The listing builds one solid part. Answer for the finished solid, in the listing's coordinates (mm). A direction names the side the tool comes from. Give positions to 0.01 mm unless a question says otherwise; leave off trailing zeros. Order: outer loops, then holes, each group sorted by start corner. A loop starts at its lowest first (then second) coordinate and runs counter-clockwise, first axis right, second up.
```python
from build123d import *

# Parameters (mm, degrees)
SKETCH1_W            = 196
SKETCH1_H            = 46
BOSS_EXTRUDE1_DEPTH  = 3.175
SKETCH2_W            = 30
SKETCH2_H            = 10.018068389
SKETCH2_W_2          = 48.596040924
SKETCH2_H_2          = 27.403064809
CUT_EXTRUDE1_DEPTH   = 3.175
M5_CLEARANCE_HOLE1_D = 5.3


with BuildPart() as part:
    # Sketch1 → Boss-Extrude1 (new body)
    with BuildSketch(Plane(origin=(0, 0, 0), x_dir=(1, 0, 0), z_dir=(0, 1, 0))):
        with Locations((98, 23)):
            Rectangle(SKETCH1_W, SKETCH1_H)
    extrude(amount=BOSS_EXTRUDE1_DEPTH)

    # Sketch2 → Cut-Extrude1 (cut)
    with BuildSketch(Plane(origin=(0, 3.175, 0), x_dir=(1, 0, 0), z_dir=(0, 1, 0))):
        with Locations((98, 40.990965805)):
            Rectangle(SKETCH2_W, SKETCH2_H)
        with BuildLine():
            ThreePointArc((83, 35.981931611), (98, 20.981931611), (113, 35.981931611))
            Line((113, 35.981931611), (83, 35.981931611))
        make_face()
        with Locations((107.298020462, 32.298467596)):
            Rectangle(SKETCH2_W_2, SKETCH2_H_2)
    extrude(amount=-CUT_EXTRUDE1_DEPTH, mode=Mode.SUBTRACT)

    # M5 Clearance Hole1 (through all)
    with Locations(Plane(origin=(0, 3.175, 0), x_dir=(1, 0, 0), z_dir=(0, 1, 0))):
        with Locations((188.5, 10), (7.5, 10), (188.5, 42), (7.5, 42)):
            Hole(M5_CLEARANCE_HOLE1_D / 2)


solid = part.part
```
1) Given P1, Ø1.6, axis at x = 114.5, y = 2.5, coming from the -Z side; P2, Ø7, axis at x = 7.5, z = -10, coming from the -Y side, each flat-ended and moving along its own axis, determine where each tip first touches the part or whether it passes through.
Geometry says:
P1: stops at z = -18.6
P2: stops at y = 0
2) Find section D-D (y = 2.15). Write down the section's boundary in (x, z), then the cut area to 3 significant figures.
Geometry says:
outline: (0, -46) - (83, -46) - (83, -18.6) - (131.6, -18.6) - (131.6, -46) - (196, -46) - (196, 0) - (0, 0) - close; hole circle Ø5.3 at (7.5, -42); hole circle Ø5.3 at (7.5, -10); hole circle Ø5.3 at (188.5, -42); hole circle Ø5.3 at (188.5, -10)
area: 7,600 mm2
3) A tool of negligible diameter and unlimited length cuts with its end or side. For faces 1 (the flat face through (0, 2, -23)), 2 (the flat face through (131.596, 2, -32)), from which of +Z, -Z, +X, -X, +Y, -Y can it reach the whole face along a straight path? Write none if from no direction.
Geometry says:
face 1: +Z, -Z, -X, +Y, -Y
face 2: -Z, +Y, -Y
4) Find section A-A (z = -37.5). Write down the section's boundary in (x, y) (3 decimals), then the cut area to 3 significant figures.
Geometry says:
outline: (0, 0) - (83, 0) - (83, 3.175) - (0, 3.175) - close; (131.596, 0) - (196, 0) - (196, 3.175) - (131.596, 3.175) - close
area: 468 mm2
5) Find section C-C (z = -10). Write down the section's boundary in (x, y) (3 decimals).
Geometry says:
outline: (0, 0) - (4.85, 0) - (4.85, 3.175) - (0, 3.175) - close; (10.15, 0) - (185.85, 0) - (185.85, 3.175) - (10.15, 3.175) - close; (191.15, 0) - (196, 0) - (196, 3.175) - (191.15, 3.175) - close
6) Straight lines are drawn through the part: probe 1 along X at (y, z) = (2.15, -42); probe 2 along Z at (x, y) = (188.5, 2.05); probe 3 along X at (y, z) = (2.45, -10). For each, find the intervals that lie inside material, in ascending order.
Geometry says:
probe 1: x = 0 to 4.85, 10.15 to 83, 131.6 to 185.85, 191.15 to 196
probe 2: z = -46 to -44.65, -39.35 to -12.65, -7.35 to 0
probe 3: x = 0 to 4.85, 10.15 to 185.85, 191.15 to 196
7) Find section B-B (x = 7.5). Write down the section's boundary in (y, z) (3 decimals).
Geometry says:
outline: (0, -46) - (3.175, -46) - (3.175, -44.65) - (0, -44.65) - close; (0, -39.35) - (3.175, -39.35) - (3.175, -12.65) - (0, -12.65) - close; (0, -7.35) - (3.175, -7.35) - (3.175, 0) - (0, 0) - close
8) For a pull along Z with two mould halves and no side action, classify faces 3 (the flat face through (41, 2, -46)), 4 (the cylindrical face through (186.05, 1.57, -8.99)), 5 (the flat face through (83, 2, -32)) as +Z half, -Z half, draft (parallel to the pull), parting line (faces both ways), or undercut.
Geometry says:
face 3: -Z half
face 4: undercut
face 5: draft
